```python
from build123d import *

# Parameters (mm, degrees)
SKETCH1_R           = 6.5
BOSS_EXTRUDE1_DEPTH = 11
SKETCH2_R           = 11
BOSS_EXTRUDE2_DEPTH = 2
FILLET1_R           = 7
DOME1_FACE_RADIUS   = 6.101020514
DOME1_HEIGHT        = 3
SKETCH3_R           = 1
CUT_EXTRUDE1_DEPTH  = 2
FILLET2_R           = 2


with BuildPart() as part:
    # Sketch1 → Boss-Extrude1 (new body)
    with BuildSketch(Plane(origin=(0, 0, 0), x_dir=(1, 0, 0), z_dir=(0, 1, 0))):
        with Locations(Location((0, 0, 0), (0, 0, 270))):
            Circle(SKETCH1_R)
    extrude(amount=BOSS_EXTRUDE1_DEPTH)

    # Sketch2 → Boss-Extrude2 (add)
    with BuildSketch(Plane.XZ):
        with Locations(Location((0, 0, 0), (0, 0, 270))):
            Circle(SKETCH2_R)
    extrude(amount=BOSS_EXTRUDE2_DEPTH)

    # Fillet1
    # the kernel refuses this fillet: 7 mm, written as the material it takes off along each edge
    with BuildSketch(Plane(origin=(0, -2, 0), x_dir=(0, 0, -1), z_dir=(-1, 0, 0))) as fillet1_piece_1:
        with BuildLine():
            CenterArc((6.101020514, -7), FILLET1_R, 45.584691403, 44.415308597)
            Line((6.101020514, 0), (6.101020514, 0.14))
            Line((6.101020514, 0.14), (11, 0.14))
            Line((11, 0.14), (11.14, 0))
            ThreePointArc((11.14, 0), (11.14, -1), (11.09797959, -1.9))
            Line((11.09797959, -1.9), (11, -2))
        make_face()
    revolve(axis=Axis((0, -2, 0), (0, -1, 0)), mode=Mode.SUBTRACT)

    # Dome1: a dome of height H over a round flat face of radius A is a cap of a sphere of radius (A * A + H * H) / (2 * H)
    dome1_r = (DOME1_FACE_RADIUS * DOME1_FACE_RADIUS + DOME1_HEIGHT * DOME1_HEIGHT) / (2 * DOME1_HEIGHT)
    dome1_base = Plane((0, -2, 0), z_dir=(0, -1, 0))
    with Locations(dome1_base.offset(DOME1_HEIGHT - dome1_r)):
        dome1_ball = Sphere(dome1_r, mode=Mode.PRIVATE)
    add(split(dome1_ball, bisect_by=dome1_base, keep=Keep.TOP, mode=Mode.PRIVATE))

    # Sketch3 → Cut-Extrude1 (cut)
    with BuildSketch(Plane(origin=(0, 0, 0), x_dir=(1, 0, 0), z_dir=(0, 1, 0))):
        with Locations(Location((-9.5, 0, 0), (0, 0, 270))):
            Circle(SKETCH3_R)
        with Locations(Location((9.5, 0, 0), (0, 0, 270))):
            Circle(SKETCH3_R)
    extrude(amount=-CUT_EXTRUDE1_DEPTH, mode=Mode.SUBTRACT)

    # Fillet2
    fillet2_edges = [part.edges().sort_by_distance(p)[0] for p in [
        (0, 11, -6.5),
    ]]
    fillet(fillet2_edges, radius=FILLET2_R)


solid = part.part
```
The model under review builds one solid part; all positions refer to its coordinate system, in mm. Round coordinates to 2 decimals unless told otherwise and drop trailing zeros. Write each loop counter-clockwise with the first axis right and the second up, starting at its lowest first coordinate (ties: lowest second). Pieces come first, ordered by that corner, then holes. Notation, with made-up numbers: (74, 42.25) - (94, 42.25) arc R12 ccw to (94, 53.25) - close; hole circle Ø6 at (-1, 47). An arc over 180 degrees is marked (long way). One line per question, with ' | ' between items.
Item 1: The part is to be moulded in two halves that separate along Z. For faces 1 (the face through (-5, 0, -5)), 2 (the face through (8.524, -0.602, -0.217)), 3 (the face through (-3.955, 4.437, -5.158)), say which applies: pulls with the +Z half, pulls with the -Z half, needs draft (parallel to the pull), parting line crosses it, or undercut.
Resolved:
face 1: needs draft | face 2: undercut | face 3: parting line crosses it
Item 2: For P1, Ø3, axis at x = 7.5, z = -8.5, coming from the +Y side; P2, Ø2.5, axis at x = -9.5, z = 0, coming from the -Y side; P3, Ø8, axis at y = 6.5, z = 0.5, coming from the +X side, all flat-tipped, find the tip position at first contact; note any pin that passes through.
Resolved:
P1: stops at y = 0 | P2: stops at y = -1.66 | P3: stops at x = 6.5
Item 3: Add section A-A, the plane y = 8. Give the boundary of the cut face in (x, z).
Resolved:
outline: circle Ø13 at (0, 0)
Item 4: To check wall thickness, follow probe 1 along X at (y, z) = (-0.25, 0); probe 2 along X at (y, z) = (-0.9, 0); probe 3 along Z at (x, y) = (4, 4.25). State the ranges of each line that lie inside material, in increasing order.
Resolved:
probe 1: x = -10.73 to -10.5, -8.5 to 8.5, 10.5 to 10.73 | probe 2: x = -8.5 to 8.5 | probe 3: z = -5.12 to 5.12
Item 5: Add section C-C, the plane y = -3. Give the boundary of the cut face in (x, z).
Resolved:
outline: circle Ø10.36 at (0, 0)
Item 6: Add section B-B, the plane z = 0. State how many separate pieces and enclosed holes the cut face has, then the cut area to 3 significant figures.
Resolved:
separate pieces: 3 | enclosed holes: 0 | area: 200 mm2
